```python
from build123d import *

# Parameters (mm, degrees)
SKETCH_1_R           = 8.5
EXTRUDE_1_DEPTH      = 2
EXTRUDE_1_2_DEPTH    = 2
EXTRUDE_7_DEPTH      = 5
EXTRUDE_7_DEPTH_BACK = 2
EXTRUDE_8_DEPTH      = 2
FILLET_1_R           = 3.8
FILLET_2_R           = 1.8
SKETCH_5_R           = 8.500000000000004
CUT_EXTRUDE_1_DEPTH  = 2
EXTRUDE_START        = 8
EXTRUDE_9_DEPTH      = 8
EXTRUDE_START_2      = 2
EXTRUDE_10_DEPTH     = 2
FILLET_3_R           = 1.8
FILLET_4_R           = 3.8
FILLET_5_R           = 2


with BuildPart() as part:
    # Sketch 1 → Extrude 1 (new body)
    with BuildSketch(Plane(origin=(0, 0, 0), x_dir=(1, 0, 0), z_dir=(0, 1, 0))):
        Polygon((0, 0), (25, 0), (39.53977757143407, 24.66022969681975), (33, 34), (0, 34), align=None)
        with Locations(Location((18, 18.000000000000004, 0), (0, 0, 270))):
            Circle(SKETCH_1_R, mode=Mode.SUBTRACT)
    extrude(amount=EXTRUDE_1_DEPTH)



with BuildPart() as body_2:
    # Sketch 1 → Extrude 1 2 (new body)
    with BuildSketch(Plane(origin=(0, 0, 0), x_dir=(1, 0, 0), z_dir=(0, 1, 0))):
        Polygon((39.539777571434044, -58.66022969681975), (32.99999999999997, -68), (-1.388e-14, -68), (-1.388e-14, -34), (24.999999999999975, -34), align=None)
        with Locations(Location((17.99999999999997, -52.00000000000001, 0), (0, 0, 90))):
            Circle(SKETCH_1_R, mode=Mode.SUBTRACT)
    extrude(amount=EXTRUDE_1_2_DEPTH)


with BuildPart() as part_1:
    add(part.part)

    add(body_2.part)  # Extrude 7 merges body 2
    # Sketch 2 → Extrude 7 (add, two sides: drawn at the far end of the back side and taken through both)
    with BuildSketch(Plane(origin=(0, 2, 0), x_dir=(1, 0, 0), z_dir=(0, 1, 0)).offset(-EXTRUDE_7_DEPTH_BACK)):
        Polygon((0, 0), (2.4e-16, -2), (26.142543519238394, -1.9999999999999973), (41.262614368883476, 23.64443770563539), (39.53977757143407, 24.66022969681975), (25, 0), align=None)
        Polygon((-1.388e-14, -34), (24.999999999999975, -34), (39.539777571434044, -58.66022969681975), (41.26261436888351, -57.644437705635355), (26.142543519238462, -32), (0, -32), align=None)
    extrude(amount=EXTRUDE_7_DEPTH + EXTRUDE_7_DEPTH_BACK)

    # Sketch 4 → Extrude 8 (add)
    with BuildSketch(Plane(origin=(0, 7, 0), x_dir=(1, 0, 0), z_dir=(0, 1, 0))):
        with BuildLine():
            Line((-1.388e-14, -34), (24.999999999999922, -34.00000000000004))
            Line((24.999999999999922, -34.00000000000004), (39.539777571434044, -58.66022969681975))
            Line((39.539777571434044, -58.66022969681975), (52.19877033120313, -51.196433079013936))
            ThreePointArc((52.19877033120313, -51.196433079013936), (37.882653193375084, -16.999999999999993), (52.19877033120313, 17.196433079013932))
            Line((52.19877033120313, 17.196433079013932), (39.539777571434044, 24.660229696819748))
            Line((39.539777571434044, 24.660229696819748), (24.999999999999982, 0))
            Line((24.999999999999982, 0), (-1.388e-14, 0))
            Line((-1.388e-14, 0), (-1.388e-14, -34))
        make_face()
    extrude(amount=EXTRUDE_8_DEPTH)

    # Fillet 1
    fillet_1_edges = [part_1.edges().sort_by_distance(p)[0] for p in [
        (33.70257894406093, 0, -10.822218852817695),
        (33.70257894406099, 0, 44.82221885281768),
        (32.26988878571699, 9, 46.33011484840989),
        (12.499999999999954, 9, 34.00000000000002),
        (32.269888785717015, 9, -12.330114848409874),
        (12.499999999999984, 9, 0),
        (13.071271759619231, 0, 32),
        (13.071271759619197, 0, 1.9999999999999987),
    ]]
    fillet(fillet_1_edges, radius=FILLET_1_R)

    # Fillet 2
    fillet_2_edges = [part_1.edges().sort_by_distance(p)[0] for p in [
        (32.269888785717036, 2, -12.330114848409876),
        (13.071271759619197, 7, 1.9999999999999987),
        (33.70257894406093, 7, -10.822218852817695),
        (32.26988878571701, 2, 46.33011484840988),
        (12.49999999999998, 2, 34),
        (33.70257894406099, 7, 44.82221885281768),
        (13.071271759619231, 7, 32),
        (12.5, 2, 0),
    ]]
    fillet(fillet_2_edges, radius=FILLET_2_R)

    # Sketch 5 → Cut-Extrude 1 (cut)
    with BuildSketch(Plane(origin=(0, 9.000000000000002, 0), x_dir=(1, 0, 0), z_dir=(0, 1, 0))):
        with Locations(Location((14.500000000000002, -17, 0), (0, 0, 270))):
            Circle(SKETCH_5_R)
    extrude(amount=-CUT_EXTRUDE_1_DEPTH, mode=Mode.SUBTRACT)

    # Sketch 6 → Extrude 9 (add)
    with BuildSketch(Plane.XZ.offset(-7).offset(EXTRUDE_START)):
        with BuildLine():
            Line((52.19877033120314, -17.19643307901394), (50.41843679588763, -18.246125394320746))
            ThreePointArc((50.41843679588763, -18.246125394320746), (35.882653193375084, 17.000000000000007), (50.41843679588763, 52.24612539432075))
            Line((50.41843679588763, 52.24612539432075), (52.19877033120313, 51.196433079013936))
            ThreePointArc((52.19877033120313, 51.196433079013936), (37.882653193375084, 16.999999999999986), (52.19877033120314, -17.19643307901394))
        make_face()
    extrude(amount=-EXTRUDE_9_DEPTH)

    # Sketch 7 → Extrude 10 (add)
    with BuildSketch(Plane.XZ.offset(1).offset(EXTRUDE_START_2)):
        with BuildLine():
            Line((50.41843679588763, 52.24612539432075), (71.4338966640132, 39.85531980164811))
            ThreePointArc((71.4338966640132, 39.85531980164811), (65.19772460662475, 17.000000000000007), (71.43389666401319, -5.8553198016480925))
            Line((71.43389666401319, -5.8553198016480925), (50.418436795887615, -18.24612539432073))
            ThreePointArc((50.418436795887615, -18.24612539432073), (35.882653193375084, 17.000000000000007), (50.41843679588763, 52.24612539432075))
        make_face()
    extrude(amount=-EXTRUDE_10_DEPTH)

    # Fillet 3
    fillet_3_edges = [part_1.edges().sort_by_distance(p)[0] for p in [
        (35.88265319337508, 7, 17.000000000000007),
        (37.88265319337509, -1, 16.999999999999996),
    ]]
    fillet(fillet_3_edges, radius=FILLET_3_R)

    # Fillet 4
    fillet_4_edges = [part_1.edges().sort_by_distance(p)[0] for p in [
        (35.88265319337508, -3, 17.000000000000014),
        (37.882653193375084, 9, 17.000000000000004),
    ]]
    fillet(fillet_4_edges, radius=FILLET_4_R)

    # Fillet 5
    fillet_5_edges = [part_1.edges().sort_by_distance(p)[0] for p in [
        (-1.388e-14, 1, 68),
        (32.99999999999997, 1, 68),
        (0, 1, -34),
        (33, 1, -34),
    ]]
    fillet(fillet_5_edges, radius=FILLET_5_R)


solid = part_1.part
```
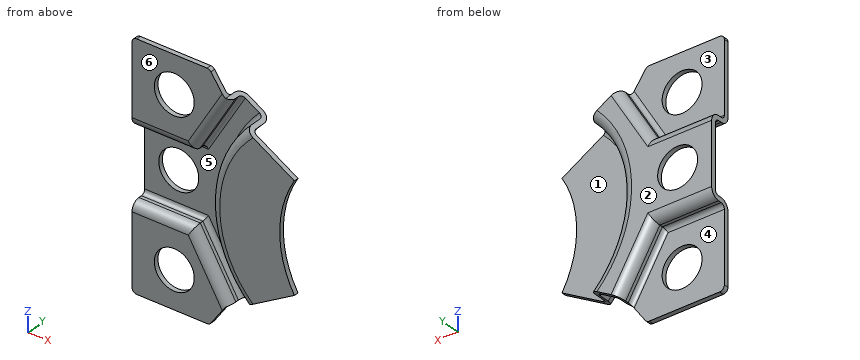
Source: CAD feature listing. Evaluate the final solid. Frame: model axes, mm. Face numbers are marked on the shaded views. A direction names the side the tool comes from. Coordinates: 2 decimals unless noted, no trailing zeros. Loops run counter-clockwise (first coordinate to the right, second up) from the corner with the lowest first, then second, coordinate; pieces in that order, holes last. Notation, with made-up numbers: (30.5, 54.25) -> (77.5, 54.25) arc R12 cw to (77.5, 65.25) -> close; hole circle Ø9 at (15, 62.25). An arc over 180 degrees is marked (long way). One line per item, written item: value. Start each with the question number.
Q1. Section query B-B, the plane x = 21.5. Give the number of separate pieces and of enclosed holes in the cut face, and give its area (3 significant figures).
Q2. Set-up query: the marked faces 1, 2, 3 and 4. Return all of +Z, -Z, +X, -X, +Y, -Y with unobstructed straight access to the full face (end or side cutting, diameter ignored); none if empty.
Q3. Contact query for flat-ended pins moving along their axis: P1, Ø9.5, axis at x = 52.5, z = 11, coming from the +Y side; P2, Ø9.5, axis at x = 14, z = 58, coming from the +Y side; P3, Ø0.7, axis at x = 12.5, y = 4.5, coming from the -Z side. Output: stop coordinate, or through.
Q4. Section query A-A, the plane z = 17. Return the cut outline in (x, y), and give its area (3 significant figures).
Q5. Mould query, pull axis X, two halves, no side actions, for the marked faces 5 and 6. Classes: pulls with the +X half, pulls with the -X half, needs draft (parallel to the pull), parting line crosses it, or undercut.
Q6. Line query: line 1 along Z through (x, y) = (20.5, 4); line 2 along X through (y, z) = (1.35, -18); line 3 along X through (y, z) = (0.75, -15.5). Output: solid intervals per line, ascending.
Results:
1. separate pieces: 4
1. enclosed holes: 0
1. area: 141 mm^2
2. face 1: +X, +Y
2. face 2: +Z, -Z, +X, -X, +Y
2. face 3: +Z, -X, +Y
2. face 4: -Z, -X, +Y
3. P1: y = -1
3. P2: y = 2
3. P3: z = 0
4. outline: (0, 7) -> (6, 7) -> (6, 9) -> (0, 9) -> close; (23, 7) -> (34.08, 7) arc R1.8 cw to (35.88, 5.2) -> (35.88, 0.8) arc R3.8 ccw to (39.68, -3) -> (65.2, -3) -> (65.2, -1) -> (39.68, -1) arc R1.8 cw to (37.88, 0.8) -> (37.88, 5.2) arc R3.8 ccw to (34.08, 9) -> (23, 9) -> close
4. area: 112 mm^2
5. face 5: undercut
5. face 6: needs draft
6. line 1: 0 to 2, 32 to 34
6. line 2: 0 to 9.5, 26.5 to 36.9, 50.18 to 50.84
6. line 3: 0 to 9.88, 26.12 to 34.68, 47.89 to 50.56
